Build history of the part. All positions in model axes, mm. A direction names the side the tool comes from. Give positions to 0.01 mm unless a question says otherwise; leave off trailing zeros. Loops run counter-clockwise (first coordinate to the right, second up) from the corner with the lowest first, then second, coordinate; pieces in that order, holes last. Notation, with made-up numbers: M -11,-17 L 37,-17 A28 cw 37,4 Z; hole C 10.5,-34 d10. An arc over 180 degrees is marked long. Answer as a JSON object with one key per item and string values. Group by question number.
1. Slice it at A-A (x = 0). List the corners of the cut face in (y, z).
2. 3-axis set-ups, long thin cutter, end or side, ignore diameter. For faces 1 (the face through (-1, -31, 0)), 2 (the face through (-0.7, -31.3, 6)): which of +Z, -Z, +X, -X, +Y, -Y reach the whole face in a straight line?
3. Mould opens along X. For faces 3 (the face through (-5.961, -26.846, 6.07)), 4 (the face through (-4.036, 30.736, 7.972)), 5 (the face through (13.2, -24.3, 11)) say: released by +X, released by -X, zero draft, split by the parting line, or undercut.
4. Drill centre lines: line 1 along Y through (x, z) = (0, 8.5); line 2 along Y through (x, z) = (0, 4.25); line 3 along Z through (x, y) = (8.5, -34). Where is each one in solid material? Low to high. Write a range as [from, to].
5. Slice it at C-C (z = 8.25). List the corners of the cut face in (x, y).
6. Drop flat-ended pins along their axis: pin 1 Ø3 at (y, z) = (-28.5, 6.5) entering from -X; pin 2 Ø12 at (x, y) = (-12.5, 10.5) entering from -Z; pin 3 Ø5 at (x, z) = (-6, 4.5) entering from +Y; pin 4 Ø1 at (y, z) = (-34, 1.5) entering from +X. Give the stop position or say it passes through.
from build123d import *

# Parameters (mm, degrees)
SCHIZZO1_R        = 48
ESTRUSIONE1_DEPTH = 6
SCHIZZO2_R        = 31
ESTRUSIONE2_DEPTH = 5
SMUSSO1_SIZE      = 1
SCHIZZO3_R        = 27.5
ESTRUSIONE3_DEPTH = 69.767724988
SMUSSO2_SIZE      = 1


with BuildPart() as part:
    # Schizzo1 → Estrusione1 (new body)
    with BuildSketch(Plane.XY):
        Circle(SCHIZZO1_R)
    extrude(amount=ESTRUSIONE1_DEPTH)

    # Schizzo2 → Estrusione2 (add)
    with BuildSketch(Plane.XY.offset(6)):
        Circle(SCHIZZO2_R)
    extrude(amount=ESTRUSIONE2_DEPTH)

    # Smusso1
    smusso1_edges = [part.edges().sort_by_distance(p)[0] for p in [
        (-48, 0, 0),
        (-31, 0, 11),
    ]]
    chamfer(smusso1_edges, length=SMUSSO1_SIZE)

    # Schizzo3 → Estrusione3 (cut, through all)
    with BuildSketch(Plane.XY.offset(11)):
        Circle(SCHIZZO3_R)
    extrude(amount=-ESTRUSIONE3_DEPTH, mode=Mode.SUBTRACT)

    # Smusso2
    smusso2_edges = [part.edges().sort_by_distance(p)[0] for p in [
        (-27.5, 0, 0),
    ]]
    chamfer(smusso2_edges, length=SMUSSO2_SIZE)


solid = part.part
Established:
{
 "1": {"outline": "M -48,1 L -47,0 L -28.5,0 L -27.5,1 L -27.5,11 L -30,11 L -31,10 L -31,6 L -48,6 Z; M 27.5,1 L 28.5,0 L 47,0 L 48,1 L 48,6 L 31,6 L 31,10 L 30,11 L 27.5,11 Z"},
 "2": {"face 1": "-Z, +X, -X, +Y, -Y", "face 2": "+Z"},
 "3": {"face 3": "undercut", "face 4": "split by the parting line", "face 5": "zero draft"},
 "4": {"line 1": "y = [-31, -27.5], [27.5, 31]", "line 2": "y = [-48, -27.5], [27.5, 48]", "line 3": "z = [0, 6]"},
 "5": {"outline": "C 0,0 d62; hole C 0,0 d55"},
 "6": {"pin 1": "stops at x = -39.63", "pin 2": "passes through", "pin 3": "stops at y = 47.87", "pin 4": "stops at x = 34.38"}
}
